from build123d import *

# Parameters (mm, degrees)
SKETCH5_R           = 7.9375
BOSS_EXTRUDE3_DEPTH = 50.8
CHAMFER1_SIZE       = 1.731818182
BOSS_EXTRUDE4_DEPTH = 10.715625
SKETCH8_OUTSIDE_W   = 256.666
SKETCH8_OUTSIDE_H   = 260.35
SKETCH8_OUTSIDE_R   = 11.90625
CUT_EXTRUDE3_DEPTH  = 62.515625
CUT_EXTRUDE3_TAPER  = 60
CUT_EXTRUDE4_DEPTH  = 0.254
CIRPATTERN1_COUNT   = 6


with BuildPart() as part:
    # Sketch5 → Boss-Extrude3 (new body)
    with BuildSketch(Plane(origin=(30.7578125, 0, 0), x_dir=(0, 0, -1), z_dir=(1, 0, 0))):
        Circle(SKETCH5_R)
    extrude(amount=-BOSS_EXTRUDE3_DEPTH)

    # Chamfer1
    chamfer1_edges = [part.edges().sort_by_distance(p)[0] for p in [
        (30.7578125, 0, 7.9375),
    ]]
    chamfer(chamfer1_edges, length=CHAMFER1_SIZE)

    # Sketch6 → Boss-Extrude4 (add)
    with BuildSketch(Plane.ZY.offset(20.0421875)):
        Polygon((11.90625, 6.874076643), (0, 13.748153285), (-11.90625, 6.874076643), (-11.90625, -6.874076643), (0, -13.748153285), (11.90625, -6.874076643), align=None)
    extrude(amount=BOSS_EXTRUDE4_DEPTH)

    # Sketch8 outside → Cut-Extrude3 (cut, through all)
    with BuildSketch(Plane.ZY.offset(30.7578125)):
        Rectangle(SKETCH8_OUTSIDE_W, SKETCH8_OUTSIDE_H)
        Circle(SKETCH8_OUTSIDE_R, mode=Mode.SUBTRACT)
    extrude(amount=-CUT_EXTRUDE3_DEPTH, taper=CUT_EXTRUDE3_TAPER, mode=Mode.SUBTRACT)

    # Sketch12 → Cut-Extrude4 (cut)
    with BuildSketch(Plane.ZY.offset(30.7578125)):
        with BuildLine():
            Line((0.3571875, 9.1678125), (0.3571875, 5.1196875))
            ThreePointArc((0.3571875, 5.1196875), (0, 4.7625), (-0.3571875, 5.1196875))
            Line((-0.3571875, 5.1196875), (-0.3571875, 9.1678125))
            ThreePointArc((-0.3571875, 9.1678125), (0, 9.525), (0.3571875, 9.1678125))
        make_face()
    cut_extrude4 = extrude(amount=-CUT_EXTRUDE4_DEPTH, mode=Mode.SUBTRACT)

    # CirPattern1: Cut-Extrude4 ×6 about axis
    cirpattern1_axis = Axis((0, 0, 0), (1, 0, 0))
    for i in range(1, CIRPATTERN1_COUNT):
        add(cut_extrude4.rotate(cirpattern1_axis, i * 360 / CIRPATTERN1_COUNT), mode=Mode.SUBTRACT)


solid = part.part
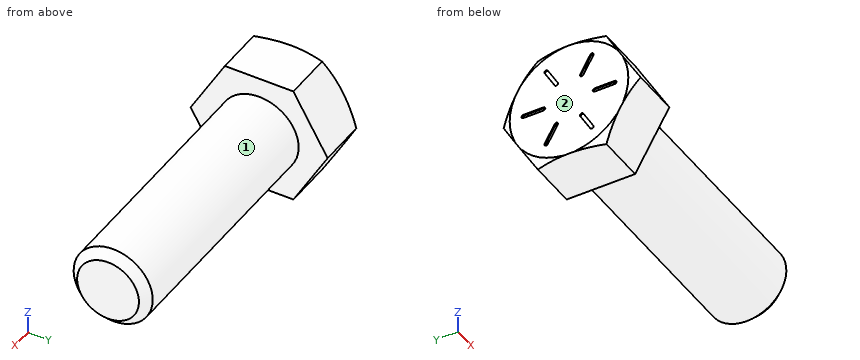
Geometry check sheet. Reference: the model listing, model coordinates, mm. Face numbers are marked on the shaded views. A direction names the side the tool comes from. Round coordinates to 2 decimals unless told otherwise and drop trailing zeros. Loops run counter-clockwise (first coordinate to the right, second up) from the corner with the lowest first, then second, coordinate; pieces in that order, holes last. Notation, with made-up numbers: (16.5, -10.5) - (37.5, -10.5) arc R5 ccw to (37.5, -3.5) - close; hole circle Ø6 at (17.5, 54.25). An arc over 180 degrees is marked (long way). One line per question, with ' | ' between items. Start each with the question number.
1. Cross-section at B-B on x = 24. Record the cut outline in (y, z) (1 decimal).
2. Cross-section at A-A on x = -21. Record the cut outline in (y, z), then the cut area to 3 significant figures.
3. Scan lines: line 1 (X direction, y = -2.25, z = 10.75); line 2 (Y direction, x = -23.5, z = 3.25); line 3 (Y direction, x = -22.5, z = -1.5). Record each from-to range of solid material in increasing order. Write a range as [from, to].
4. Tool access check on the marked faces 1 and 2. Record the directions out of +Z, -Z, +X, -X, +Y, -Y that give a thin tool (end or side, any length) a straight path to the whole face; none if there is none.
5. Depth check by flat-ended pin: pin 1 (0.6 mm diameter, centred on y = 7, z = 0, fed in from -X); pin 2 (3 mm diameter, centred on x = -16.5, z = 8.5, fed in from +Y); pin 3 (2 mm diameter, centred on x = 7, z = 7, fed in from +Y). Enter the tip coordinate at first touch or a pass-through.
Taken from the geometry:
1) outline: circle Ø15.9 at (0, 0)
2) outline: (-13.75, 0) - (-6.87, -11.91) - (6.87, -11.91) - (13.75, 0) - (6.87, 11.91) - (-6.87, 11.91) - close | area: 491 mm²
3) line 1: [-30.76, -20.04] | line 2: [-11.87, 11.87] | line 3: [-12.88, 12.88]
4) face 1: +X | face 2: +Z, -Z, -X, +Y, -Y
5) pin 1: x = -30.5 | pin 2: y = 3.74 | pin 3: y = 5.2
